Read the model definition and answer for the solid it produces. Units are mm, in the model's axes. A direction names the side the tool comes from. Round coordinates to 2 decimals unless told otherwise and drop trailing zeros. Write each loop counter-clockwise with the first axis right and the second up, starting at its lowest first coordinate (ties: lowest second). Pieces come first, ordered by that corner, then holes. Notation, with made-up numbers: (28, -13.75) -> (79, -13.75) arc R38 ccw to (79, 25.25) -> close; hole circle Ø10 at (43, -32). An arc over 180 degrees is marked (long way). Return JSON: item names as keys, results as strings. Group by question number.
(1) A cutting plane is placed at A-A on z = 52. Give the vertices of the cut face in (x, y).
(2) A cutting plane is placed at C-C on y = 10.5. Give the vertices of the cut face in (x, z), then the cut area to 3 significant figures.
(3) For faces 1 (the flat face through (-2, 23, 0)), 2 (the flat face through (31.151, 6, 44)), 3 (the flat face through (-10, 18, 3)), determine the directions among +Z, -Z, +X, -X, +Y, -Y from which every point of the face is accessible in a straight line to the end or side of a thin tool.
(4) A cutting plane is placed at D-D on x = 13. Give the vertices of the cut face in (y, z).
(5) A cutting plane is placed at B-B on y = 3.5. Give the vertices of the cut face in (x, z), then the cut area to 3 significant figures.
(6) Straight lines are drawn through the part: line 1 (Z direction, x = 13.5, y = 25.5); line 2 (X direction, y = 26, z = 12); line 3 (Y direction, x = 17, z = 6). For each, find the intervals that lie inside material, in ascending order.
(7) Given pin 1 (8 mm diameter, centred on y = 12.5, z = 23, fed in from +X); pin 2 (7.5 mm diameter, centred on y = 11.5, z = 53.5, fed in from -X); pin 3 (18.5 mm diameter, centred on y = 11.5, z = 28.5, fed in from -X), each flat-ended and moving along its own axis, determine where each tip first touches the part or whether it passes through.
(8) The mould has two halves that part along Y. Classify faces 4 (the flat face through (39, 0, 46)), 5 (the cylindrical face through (-11.434, 3.728, 1.479)), 6 (the flat face through (11.151, 6, 44)): released by +Y, released by -Y, zero draft, split by the parting line, or undercut.
Autodesk Inventor part; units mm, degrees
ref_plane "YZ Plane" through (0, 0, 0) normal (1, 0, 0) x (0, 1, 0)
ref_plane "XZ Plane" through (0, 0, 0) normal (0, 1, 0) x (-1, 0, 0)
ref_plane "XY Plane" through (0, 0, 0) normal (0, 0, 1) x (1, 0, 0)
sketch "Boceto1" plane through (0, 0, 0) normal (0, 0, 1) x (1, 0, 0)
  line L0 (42.301, 0) -> (42.301, 9.6)
  line L1 (42.302, 9.6) -> (42.302, 26.1)
  line L2 (42.301, 26.1) -> (42.301, 33.75)
  line L3 (38.301, 0) -> (42.301, 0)
  line L4 (4.001, 33.75) -> (38.301, 33.75)
  line L5 (38.301, 33.75) -> (42.301, 33.75)
  line L6 (0.001, 33.75) -> (4.001, 33.75)
  line L7 (0.001, 26.1) -> (0.001, 33.75)
  line L8 (0.001, 9.6) -> (0.001, 26.1)
  line L9 (0.001, 0) -> (0.001, 9.6)
  line L10 (42.301, 33.75) -> (0.001, 33.75)
  line L11 (0.001, 33.75) -> (0.001, 0)
  line L12 (0.001, 0) -> (42.301, 0)
  line L13 (42.301, 0) -> (42.301, 33.75)
  line L14 (42.501, 33.95) -> (-0.199, 33.95)
  line L15 (-0.199, 33.95) -> (-0.199, -0.2)
  line L16 (-0.199, -0.2) -> (42.501, -0.2)
  line L17 (42.501, -0.2) -> (42.501, 33.95)
  line L18 (42.501, 36.95) -> (-3.199, 36.95)
  line L19 (-3.199, 36.95) -> (-3.199, 0)
  line L20 (-3.199, -3.2) -> (45.501, -3.2)
  line L21 (45.501, 0) -> (45.501, 36.95)
  line L22 (42.301, 0) -> (45.501, 0)
  line L23 (0.001, 0) -> (-3.199, 0)
  line L24 (42.501, 33.95) -> (42.501, 36.95)
  point P0 (0, 0)
  point P1 (-0.199, 0)
  dimension "d0" = 0.2
  dimension "d1" = 3
extrude "Extrusión1" add sketch "Boceto1" along normal blind 45.502 contours L14 L15 L23 L19 L18 L24
sketch "Boceto2" plane through (-0.199, 33.95, 0) normal (0, -1, 0) x (1, 0, 0)
  line L0 (0, 0) -> (42.7, 0)
  line L1 (42.7, 0) -> (42.7, 45.502)
  line L2 (0, 45.502) -> (42.7, 45.502)
  line L3 (0, 0) -> (0, 45.502)
  line L4 (42.7, 45.502) -> (0, 45.502)
  line L5 (0, 45.502) -> (0, 42.502)
  line L6 (0, 42.502) -> (42.7, 42.502)
  line L7 (42.7, 42.502) -> (42.7, 45.502)
  point P0 (0.199, 0)
  dimension "d4" = 3
extrude "Extrusión2" add sketch "Boceto2" along normal up to surface (33.95 mm away) contours L3 L2 L1 L6
sketch "Boceto3" plane through (0, 0, 45.502) normal (0, 0, 1) x (1, 0, 0)
  line L0 (-3.199, 0) -> (42.501, 0)
  line L1 (42.501, 36.95) -> (42.501, 0)
  line L2 (42.501, 36.95) -> (-3.199, 36.95)
  line L3 (-3.199, 36.95) -> (-3.199, 0)
  line L4 (-6.5037, 43.25) -> (-6.5037, 58.25)
  line L5 (-6.5037, 43.25) -> (-6.5037, 58.25)
  line L6 (29.151, 9.6) -> (29.151, 3.2)
  line L7 (29.151, 0) -> (29.151, 3.2)
  line L8 (13.651, 3.6) -> (13.651, 9.1)
  line L9 (13.151, 3.2) -> (13.151, 0)
  line L10 (13.151, 9.6) -> (13.151, 3.2)
  line L11 (29.151, 9.6) -> (13.151, 9.6)
  line L12 (11.151, 0) -> (11.151, 3.2)
  line L13 (11.151, 3.2) -> (11.151, 11.6)
  line L14 (11.151, 11.6) -> (31.151, 11.6)
  line L15 (31.151, 11.6) -> (31.151, 3.2)
  line L16 (31.151, 3.2) -> (31.151, 0)
  point P0 (0, 0)
  point P1 (-15.9908, 43.25)
  dimension "d7" = 2
extrude "Extrusión3" cut sketch "Boceto3" against normal blind 10 contours L12 L13 L14 L15 L16 L0 L7 L6 L11 L10 L9 | L9 L10 L11 L6 L7 L0
sketch "Boceto4" plane through (-3.199, 36.95, 0) normal (0, 1, 0) x (1, 0, 0)
  circle A0 centre (24.35, -21.151) radius 2.5
  circle A1 centre (24.35, -21.151) radius 15
  point P0 (3.199, 0)
  dimension "d10" = 30
extrude "Extrusión4" cut sketch "Boceto4" against normal blind 10 contours A0 | A1
sketch "Boceto5" plane through (-3.199, 36.95, 0) normal (0, 1, 0) x (1, 0, 0)
  circle A0 centre (24.35, -21.151) radius 15
  line L0 (45.7, 0) -> (0, 0)
  line L1 (0, 0) -> (0, -45.502)
  line L2 (45.7, -45.502) -> (0, -45.502)
  line L3 (45.7, 0) -> (45.7, -45.502)
  circle A1 centre (24.35, -21.151) radius 15
  line L4 (45.7, -42.502) -> (3, -42.502)
  line L5 (3, 0) -> (3, -42.502)
  line L6 (3, 0) -> (45.7, 0)
  line L7 (45.7, 0) -> (45.7, -42.502)
  circle A2 centre (8.85, -36.651) radius 1.5
  circle A3 centre (8.85, -5.651) radius 1.5
  circle A4 centre (39.85, -5.6509) radius 1.5001
  circle A5 centre (39.8499, -36.6509) radius 1.4998
  circle A6 centre (39.8499, -36.6509) radius 2
  circle A7 centre (39.85, -5.6509) radius 2
  circle A8 centre (8.85, -5.651) radius 2
  circle A9 centre (8.85, -36.651) radius 2
  point P0 (3.199, 0)
  dimension "d13" = 4
  dimension "d14" = 4
  dimension "d15" = 4
  dimension "d16" = 4
hole "Agujero1" at (5.651, 36.95, 36.651) at (5.651, 36.95, 5.651) at (36.651, 36.95, 5.6509) at (36.6509, 36.95, 36.6509) direction (0, -1, 0) diameter 3.5 end through all
sketch "Boceto6" plane through (0, 0, 45.502) normal (0, 0, 1) x (1, 0, 0)
  line L0 (31.151, 11.6) -> (31.151, 0)
  line L1 (31.151, 0) -> (42.501, 0)
  line L2 (42.501, 36.95) -> (42.501, 0)
  line L3 (42.501, 36.95) -> (-3.199, 36.95)
  line L4 (-3.199, 36.95) -> (-3.199, 0)
  line L5 (-3.199, 0) -> (11.151, 0)
  line L6 (11.151, 0) -> (11.151, 11.6)
  line L7 (11.151, 11.6) -> (31.151, 11.6)
  line L8 (42.501, 36.95) -> (39.501, 36.95)
  line L9 (39.501, 36.95) -> (39.501, 0)
  line L10 (39.501, 0) -> (42.501, 0)
  line L11 (42.501, 0) -> (42.501, 36.95)
  point P0 (0, 0)
  dimension "d24" = 3
extrude "Extrusión5" add sketch "Boceto6" along normal blind 10 contours L9 L3 L2 L1
fillet "Empalme1" radius 3 1 edges at (39.501, 18.475, 45.502)
sketch "Boceto7" plane through (39.501, 0, 55.502) normal (-1, 0, 0) x (0, 0, 1)
  line L0 (-7, 0) -> (-7, 36.95)
  line L1 (-7, 0) -> (0, 0)
  line L2 (0, 36.95) -> (0, 0)
  line L3 (-7, 36.95) -> (0, 36.95)
  line L4 (-7, 36.95) -> (0, 36.95)
  line L5 (0, 36.95) -> (0, 29.95)
  line L6 (0, 29.95) -> (-7, 29.95)
  line L7 (-7, 29.95) -> (-7, 36.95)
  line L8 (-55.502, 36.95) -> (0, 36.95)
  line L9 (-7, 29.95) -> (0, 36.95)
  circle A0 centre (-3.5, 33.45) radius 2
  line L10 (-7, 0) -> (0, 0)
  line L11 (0, 0) -> (0, 7)
  line L12 (0, 7) -> (-7, 7)
  line L13 (-7, 7) -> (-7, 0)
  line L14 (-7, 0) -> (0, 7)
  circle A1 centre (-3.5, 3.5) radius 2
  point P0 (-55.502, 0)
  dimension "d28" = 7
  dimension "d29" = 4
  dimension "d30" = 7
  dimension "d31" = 7
  dimension "d32" = 4
hole "Agujero2" at (39.501, 33.45, 52.002) at (39.501, 3.5, 52.002) direction (1, 0, 0) diameter 3.5 end through all
sketch "Boceto8" plane through (-3.199, 0, 0) normal (-1, 0, 0) x (0, 0, 1)
  line L0 (0, 36.95) -> (0, 0)
  line L1 (0, 0) -> (45.502, 0)
  line L2 (45.502, 36.95) -> (45.502, 0)
  line L3 (0, 36.95) -> (45.502, 36.95)
  line L4 (0, 0) -> (3, 0)
  line L5 (3, 0) -> (3, 36.95)
  line L6 (3, 36.95) -> (0, 36.95)
  line L7 (0, 36.95) -> (0, 0)
  point P0 (0, 0)
  dimension "d40" = 3
extrude "Extrusión6" add sketch "Boceto8" along normal blind 10 contours L3 L5 L1 L0
fillet "Empalme2" radius 3 1 edges at (-3.199, 18.475, 3)
sketch "Boceto9" plane through (-13.199, 0, 3) normal (0, 0, 1) x (1, 0, 0)
  line L0 (7, 36.95) -> (7, 0)
  line L1 (7, 36.95) -> (0, 36.95)
  line L2 (0, 0) -> (0, 36.95)
  line L3 (7, 0) -> (0, 0)
  line L4 (0, 36.95) -> (7, 36.95)
  line L5 (7, 36.95) -> (7, 29.95)
  line L6 (7, 29.95) -> (0, 29.95)
  line L7 (0, 29.95) -> (0, 36.95)
  line L8 (0, 0) -> (7, 0)
  line L9 (7, 0) -> (7, 7)
  line L10 (7, 7) -> (0, 7)
  line L11 (0, 7) -> (0, 0)
  line L12 (0, 29.95) -> (7, 36.95)
  line L13 (0, 7) -> (7, 0)
  circle A0 centre (3.5, 33.45) radius 1.75
  circle A1 centre (3.5, 3.5) radius 1.75
  point P0 (13.199, 0)
  dimension "d44" = 7
  dimension "d45" = 7
  dimension "d46" = 7
  dimension "d47" = 3.5
  dimension "d48" = 3.5
hole "Agujero3" at (-9.699, 33.45, 3) at (-9.699, 3.5, 3) direction (0, 0, -1) diameter 3.5 end through all
fillet "Empalme3" radius 3 1 edges at (-3.199, 18.475, 45.502)
properties part number "Soporte Motor"
Checks:
{
 "1": {"outline": "(39.5, 0) -> (42.5, 0) -> (42.5, 1.75) -> (39.5, 1.75) -> close; (39.5, 5.25) -> (42.5, 5.25) -> (42.5, 31.7) -> (39.5, 31.7) -> close; (39.5, 35.2) -> (42.5, 35.2) -> (42.5, 36.95) -> (39.5, 36.95) -> close"},
 "2": {"outline": "(-13.2, 0) -> (-0.2, 0) -> (-0.2, 42.5) -> (11.15, 42.5) -> (11.15, 45.5) -> (-0.2, 45.5) arc R3 ccw to (-3.2, 42.5) -> (-3.2, 6) arc R3 cw to (-6.2, 3) -> (-13.2, 3) -> close; (31.15, 42.5) -> (42.5, 42.5) -> (42.5, 55.5) -> (39.5, 55.5) -> (39.5, 48.5) arc R3 cw to (36.5, 45.5) -> (31.15, 45.5) -> close", "area": "267 mm^2"},
 "3": {"face 1": "-Z, +X, -X, +Y, -Y", "face 2": "+Z, -Z, -Y", "face 3": "+Z, -X, +Y, -Y"},
 "4": {"outline": "(11.6, 42.5) -> (33.95, 42.5) -> (33.95, 33.74) -> (36.95, 33.74) -> (36.95, 45.5) -> (11.6, 45.5) -> close; (33.95, 0) -> (36.95, 0) -> (36.95, 8.56) -> (33.95, 8.56) -> close"},
 "5": {"outline": "(-13.2, 0) -> (-11.45, 0) -> (-11.45, 3) -> (-13.2, 3) -> close; (-7.95, 0) -> (-0.2, 0) -> (-0.2, 42.5) -> (11.15, 42.5) -> (11.15, 45.5) -> (-0.2, 45.5) arc R3 ccw to (-3.2, 42.5) -> (-3.2, 6) arc R3 cw to (-6.2, 3) -> (-7.95, 3) -> close; (31.15, 42.5) -> (42.5, 42.5) -> (42.5, 50.25) -> (39.5, 50.25) -> (39.5, 48.5) arc R3 cw to (36.5, 45.5) -> (31.15, 45.5) -> close; (39.5, 53.75) -> (42.5, 53.75) -> (42.5, 55.5) -> (39.5, 55.5) -> close", "area": "246 mm^2"},
 "6": {"line 1": "z = 42.5 to 45.5", "line 2": "x = -3.2 to -0.2", "line 3": "y = 33.95 to 36.95"},
 "7": {"pin 1": "stops at x = -0.2", "pin 2": "stops at x = 39.5", "pin 3": "stops at x = -3.2"},
 "8": {"face 4": "released by -Y", "face 5": "undercut", "face 6": "zero draft"}
}
